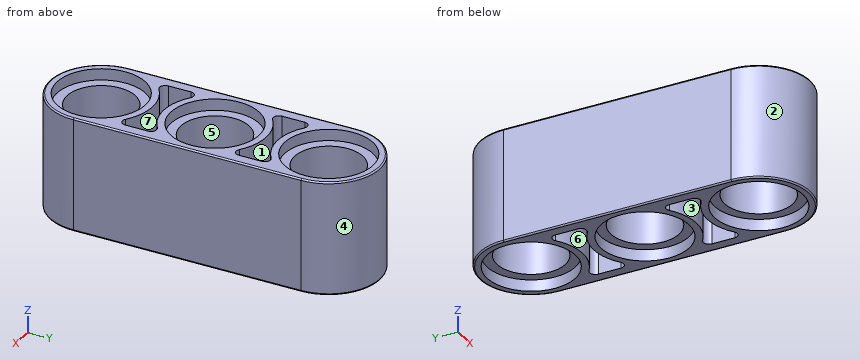
```python
from build123d import *

# Parameters (mm, degrees)
BOSS_EXTRUDE1_DEPTH = 8
CUT_EXTRUDE2_DEPTH  = 3.1
CUT_EXTRUDE4_DEPTH  = 3.1
CUT_EXTRUDE6_DEPTH  = 3.1
CUT_EXTRUDE7_DEPTH  = 3.1
FILLET1_R           = 0.1


with BuildPart() as part:
    # Sketch1 → Boss-Extrude1 (new body)
    with BuildSketch(Plane.XY.offset(4)):
        with BuildLine():
            Line((-3.6, 0), (-3.6, -16))
            ThreePointArc((-3.6, -16), (0, -19.6), (3.6, -16))
            Line((3.6, -16), (3.6, 0))
            ThreePointArc((3.6, 0), (0, 3.6), (-3.6, 0))
        make_face()
    extrude(amount=-BOSS_EXTRUDE1_DEPTH)

    # Sketch3 → Cut-Extrude2 (cut)
    with BuildSketch(Plane.XY.offset(4)):
        with BuildLine():
            Line((2.8, -4.8), (2.8, -3.2))
            ThreePointArc((2.8, -3.2), (2.578885438, -2.842229124), (2.16, -2.88))
            ThreePointArc((2.16, -2.88), (0, -3.6), (-2.16, -2.88))
            ThreePointArc((-2.16, -2.88), (-2.578885438, -2.842229124), (-2.8, -3.2))
            Line((-2.8, -3.2), (-2.8, -4.8))
            ThreePointArc((-2.8, -4.8), (-2.578885438, -5.157770876), (-2.16, -5.12))
            ThreePointArc((-2.16, -5.12), (0, -4.4), (2.16, -5.12))
            ThreePointArc((2.16, -5.12), (2.578885438, -5.157770876), (2.8, -4.8))
        make_face()
    extrude(amount=-CUT_EXTRUDE2_DEPTH, mode=Mode.SUBTRACT)

    # Sketch5 → Cut-Extrude4 (cut)
    with BuildSketch(Plane.XY.offset(4)):
        with BuildLine():
            Line((2.8, -12.8), (2.8, -11.2))
            ThreePointArc((2.8, -11.2), (2.578885438, -10.842229124), (2.16, -10.88))
            ThreePointArc((2.16, -10.88), (0, -11.6), (-2.16, -10.88))
            ThreePointArc((-2.16, -10.88), (-2.578885438, -10.842229124), (-2.8, -11.2))
            Line((-2.8, -11.2), (-2.8, -12.8))
            ThreePointArc((-2.8, -12.8), (-2.578885438, -13.157770876), (-2.16, -13.12))
            ThreePointArc((-2.16, -13.12), (0, -12.4), (2.16, -13.12))
            ThreePointArc((2.16, -13.12), (2.578885438, -13.157770876), (2.8, -12.8))
        make_face()
    extrude(amount=-CUT_EXTRUDE4_DEPTH, mode=Mode.SUBTRACT)

    # Sketch7 → Cut-Extrude6 (cut)
    with BuildSketch(Plane(origin=(0, 0, -4), x_dir=(-1, 0, 0), z_dir=(0, 0, -1))):
        with BuildLine():
            Line((2.8, -4.8), (2.8, -3.2))
            ThreePointArc((2.8, -3.2), (2.578885438, -2.842229124), (2.16, -2.88))
            ThreePointArc((2.16, -2.88), (0, -3.6), (-2.16, -2.88))
            ThreePointArc((-2.16, -2.88), (-2.578885438, -2.842229124), (-2.8, -3.2))
            Line((-2.8, -3.2), (-2.8, -4.8))
            ThreePointArc((-2.8, -4.8), (-2.578885438, -5.157770876), (-2.16, -5.12))
            ThreePointArc((-2.16, -5.12), (0, -4.4), (2.16, -5.12))
            ThreePointArc((2.16, -5.12), (2.578885438, -5.157770876), (2.8, -4.8))
        make_face()
    extrude(amount=-CUT_EXTRUDE6_DEPTH, mode=Mode.SUBTRACT)

    # Sketch8 → Cut-Extrude7 (cut)
    with BuildSketch(Plane(origin=(0, 0, -4), x_dir=(-1, 0, 0), z_dir=(0, 0, -1))):
        with BuildLine():
            Line((-2.8, -11.2), (-2.8, -12.8))
            ThreePointArc((-2.8, -12.8), (-2.578885438, -13.157770876), (-2.16, -13.12))
            ThreePointArc((-2.16, -13.12), (0, -12.4), (2.16, -13.12))
            ThreePointArc((2.16, -13.12), (2.578885438, -13.157770876), (2.8, -12.8))
            Line((2.8, -12.8), (2.8, -11.2))
            ThreePointArc((2.8, -11.2), (2.578885438, -10.842229124), (2.16, -10.88))
            ThreePointArc((2.16, -10.88), (0, -11.6), (-2.16, -10.88))
            ThreePointArc((-2.16, -10.88), (-2.578885438, -10.842229124), (-2.8, -11.2))
        make_face()
    extrude(amount=-CUT_EXTRUDE7_DEPTH, mode=Mode.SUBTRACT)

    # Sketch10 → Cut-Revolve1 (revolve, cut)
    with BuildSketch(Plane(origin=(0, -16, 0), x_dir=(1, 0, 0), z_dir=(0, 1, 0))):
        Polygon((3.1, 4), (0, 4), (0, -4), (3.1, -4), (3.1, -3.2), (2.4, -3.2), (2.4, 3.2), (3.1, 3.2), align=None)
    revolve(axis=Axis((0, -16, -4), (0, 0, 1)), mode=Mode.SUBTRACT)

    # Sketch12 → Cut-Revolve3 (revolve, cut)
    with BuildSketch(Plane(origin=(0, -8, 0), x_dir=(1, 0, 0), z_dir=(0, 1, 0))):
        Polygon((3.1, 4), (0, 4), (0, -4), (3.1, -4), (3.1, -3.2), (2.4, -3.2), (2.4, 3.2), (3.1, 3.2), align=None)
    revolve(axis=Axis((0, -8, -4), (0, 0, 1)), mode=Mode.SUBTRACT)

    # Sketch13 → Cut-Revolve4 (revolve, cut)
    with BuildSketch(Plane(origin=(0, 0, 0), x_dir=(1, 0, 0), z_dir=(0, 1, 0))):
        Polygon((3.1, 4), (0, 4), (0, -4), (3.1, -4), (3.1, -3.2), (2.4, -3.2), (2.4, 3.2), (3.1, 3.2), align=None)
    revolve(axis=Axis((0, 0, -4), (0, 0, 1)), mode=Mode.SUBTRACT)

    # Fillet1
    fillet1_edges = [part.edges().sort_by_distance(p)[0] for p in [
        (0, -19.6, -4),
        (3.6, -8, -4),
        (0, 3.6, -4),
        (3.6, -8, 4),
        (0, -19.6, 4),
        (-3.6, -8, 4),
        (0, 3.6, 4),
        (-3.6, -8, -4),
    ]]
    fillet(fillet1_edges, radius=FILLET1_R)


solid = part.part
```
Input: part model. Units: mm. Frame: model coordinates. Face numbers are marked on the shaded views. A direction names the side the tool comes from. Coordinates: 2 decimals unless noted, no trailing zeros. Loops run counter-clockwise (first coordinate to the right, second up) from the corner with the lowest first, then second, coordinate; pieces in that order, holes last.
Q1. Contact query for flat-ended pins moving along their axis: pin 1 (3 mm diameter, centred on x = 0, y = 0, fed in from -Z); pin 2 (3 mm diameter, centred on x = -1, y = -1, fed in from -Z). Output: stop coordinate, or through.
Results are:
pin 1: passes through
pin 2: stops at z = -3.2
Q2. Mould query, pull axis Y, two halves, no side actions, for the marked faces 1, 2, 3 and 4. Classes: +Y half, -Y half, draft (parallel to the pull), parting line (faces both ways), or undercut.
Results are:
face 1: undercut
face 2: -Y half
face 3: undercut
face 4: +Y half
Q3. Line query: line 1 along Y through (x, z) = (0, -3.75); line 2 along Y through (x, z) = (0, 0); line 3 along Y through (x, z) = (0, -1). Output: solid intervals per line, ascending.
Results are:
line 1: y = -19.6 to -19.1, -12.9 to -12.4, -11.6 to -11.1, -4.9 to -4.4, -3.6 to -3.1, 3.1 to 3.6
line 2: y = -19.6 to -18.4, -13.6 to -10.4, -5.6 to -2.4, 2.4 to 3.6
line 3: y = -19.6 to -18.4, -13.6 to -12.4, -11.6 to -10.4, -5.6 to -4.4, -3.6 to -2.4, 2.4 to 3.6
Q4. Section A-A, the plane y = -8.75. Return the cut outline in (x, z).
Results are:
outline: (-3.6, -3.9) arc R0.1 ccw to (-3.5, -4) - (-3.01, -4) - (-3.01, -3.2) - (-2.28, -3.2) - (-2.28, 3.2) - (-3.01, 3.2) - (-3.01, 4) - (-3.5, 4) arc R0.1 ccw to (-3.6, 3.9) - close; (2.28, -3.2) - (3.01, -3.2) - (3.01, -4) - (3.5, -4) arc R0.1 ccw to (3.6, -3.9) - (3.6, 3.9) arc R0.1 ccw to (3.5, 4) - (3.01, 4) - (3.01, 3.2) - (2.28, 3.2) - close
Q5. Section B-B, the plane z = -2.75. Return the cut outline in (x, y).
Results are:
outline: (-3.6, -16) arc R3.6 ccw to (3.6, -16) - (3.6, 0) arc R3.6 ccw to (-3.6, 0) - close; hole (-2.8, -12.8) arc R0.4 ccw to (-2.16, -13.12) arc R3.6 cw to (2.16, -13.12) arc R0.4 ccw to (2.8, -12.8) - (2.8, -11.2) arc R0.4 ccw to (2.16, -10.88) arc R3.6 cw to (-2.16, -10.88) arc R0.4 ccw to (-2.8, -11.2) - close; hole (-2.8, -4.8) arc R0.4 ccw to (-2.16, -5.12) arc R3.6 cw to (2.16, -5.12) arc R0.4 ccw to (2.8, -4.8) - (2.8, -3.2) arc R0.4 ccw to (2.16, -2.88) arc R3.6 cw to (-2.16, -2.88) arc R0.4 ccw to (-2.8, -3.2) - close; hole circle Ø4.8 at (0, -16); hole circle Ø4.8 at (0, -8); hole circle Ø4.8 at (0, 0)
Q6. Section D-D, the plane y = -12. Return the cut outline in (x, z).
Results are:
outline: (-3.6, -3.9) arc R0.1 ccw to (-3.5, -4) - (-2.8, -4) - (-2.8, -0.9) - (2.8, -0.9) - (2.8, -4) - (3.5, -4) arc R0.1 ccw to (3.6, -3.9) - (3.6, 3.9) arc R0.1 ccw to (3.5, 4) - (2.8, 4) - (2.8, 0.9) - (-2.8, 0.9) - (-2.8, 4) - (-3.5, 4) arc R0.1 ccw to (-3.6, 3.9) - close
Q7. Section C-C, the plane x = 0. Give the number of separate pieces and of enclosed holes in the cut face, and give its area (3 significant figures).
Results are:
separate pieces: 4
enclosed holes: 0
area: 53.8 mm2
Q8. Set-up query: the marked faces 5, 6 and 7. Return all of +Z, -Z, +X, -X, +Y, -Y with unobstructed straight access to the full face (end or side cutting, diameter ignored); none if empty.
Results are:
face 5: +Z, -Z
face 6: -Z
face 7: +Z
